Check sheet for the modelled part. Datum: model origin and axes. Units: mm. Face numbers are marked on the shaded views. A direction names the side the tool comes from. Round coordinates to 2 decimals unless told otherwise and drop trailing zeros. Write each loop counter-clockwise with the first axis right and the second up, starting at its lowest first coordinate (ties: lowest second). Pieces come first, ordered by that corner, then holes. Notation, with made-up numbers: (77, -28.5) -> (128, -28.5) arc R6 cw to (128, -17.5) -> close; hole circle Ø7 at (-38, -39). An arc over 180 degrees is marked (long way). Write item = value, one per line.
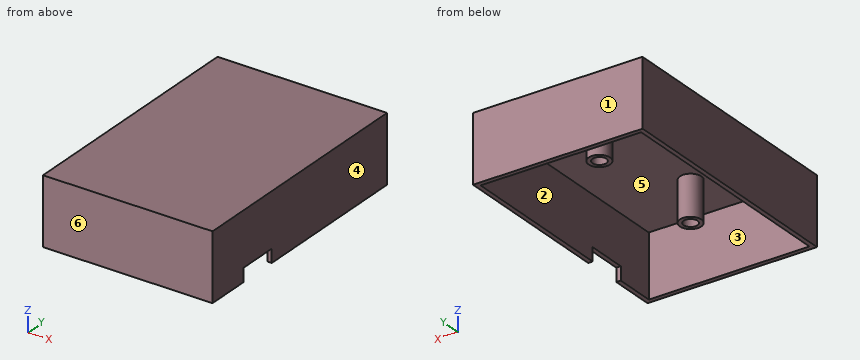
from build123d import *

# Parameters (mm, degrees)
SKETCH030_W     = 38
SKETCH030_H     = 56
PAD017_DEPTH    = 15
SKETCH031_W     = 36
SKETCH031_H     = 54
POCKET007_DEPTH = 14
SKETCH033_R     = 2.4
SKETCH033_R_2   = 1.55
PAD019_DEPTH    = 9
SKETCH038_W     = 9
SKETCH038_H     = 3
POCKET010_DEPTH = 5


with BuildPart() as part:
    # Sketch030 → Pad017 (new body)
    with BuildSketch(Plane.XY):
        Rectangle(SKETCH030_W, SKETCH030_H)
    extrude(amount=PAD017_DEPTH)

    # Sketch031 (on Face5 of Pad017) → Pocket007 (cut)
    with BuildSketch(Plane(origin=(0, 0, 0), x_dir=(1, 0, 0), z_dir=(0, 0, -1))):
        Rectangle(SKETCH031_W, SKETCH031_H)
    extrude(amount=-POCKET007_DEPTH, mode=Mode.SUBTRACT)

    # Sketch033 (on Face11 of Pocket007) → Pad019 (join)
    with BuildSketch(Plane(origin=(0, 0, 14), x_dir=(1, 0, 0), z_dir=(0, 0, -1))):
        with Locations((0, 14.65)):
            Circle(SKETCH033_R)
        with Locations((0, 14.65)):
            Circle(SKETCH033_R_2, mode=Mode.SUBTRACT)
    pad019 = extrude(amount=PAD019_DEPTH)

    # Mirrored009: Pad019 across XZ
    add(pad019.mirror(Plane.XZ))

    # Sketch038 (on Face3 of Mirrored009) → Pocket010 (cut)
    with BuildSketch(Plane.YZ.offset(19)):
        with Locations((-13.5, 1.5)):
            Rectangle(SKETCH038_W, SKETCH038_H)
    extrude(amount=-POCKET010_DEPTH, mode=Mode.SUBTRACT)


with BuildPart() as part_1:
    # Body007 placement: moved
    add(part.part.moved(Location((0, 0, 6.6))))


solid = part_1.part
(1) Release check for a two-part mould opening along X. For the marked faces 3, 4, 5 and 6 record: pulls with the +X half, pulls with the -X half, needs draft (parallel to the pull), parting line crosses it, or undercut.
Worked answers:
face_3 = undercut
face_4 = pulls with the +X half
face_5 = undercut
face_6 = needs draft
(2) Sectioned sample at D-D on x = 0. Enter the section's corners in (y, z).
Worked answers:
outline = (-28, 6.6) -> (-27, 6.6) -> (-27, 20.6) -> (-17.05, 20.6) -> (-17.05, 11.6) -> (-16.2, 11.6) -> (-16.2, 20.6) -> (-13.1, 20.6) -> (-13.1, 11.6) -> (-12.25, 11.6) -> (-12.25, 20.6) -> (12.25, 20.6) -> (12.25, 11.6) -> (13.1, 11.6) -> (13.1, 20.6) -> (16.2, 20.6) -> (16.2, 11.6) -> (17.05, 11.6) -> (17.05, 20.6) -> (27, 20.6) -> (27, 6.6) -> (28, 6.6) -> (28, 21.6) -> (-28, 21.6) -> close
(3) Sectioned sample at B-B on y = -10.5. Enter the section's corners in (x, z).
Worked answers:
outline = (-19, 6.6) -> (-18, 6.6) -> (-18, 20.6) -> (18, 20.6) -> (18, 9.6) -> (19, 9.6) -> (19, 21.6) -> (-19, 21.6) -> close
(4) Material ranges on L1, parallel to Y at x = 0, z = 14.5; L2, parallel to X at y = -14.65, z = 15.5; L3, parallel to Y at x = 2.5, z = 12.25, recorded low to high. Write a range as [from, to].
Worked answers:
L1 = [-28, -27], [-17.05, -16.2], [-13.1, -12.25], [12.25, 13.1], [16.2, 17.05], [27, 28]
L2 = [-19, -18], [-2.4, -1.55], [1.55, 2.4], [18, 19]
L3 = [-28, -27], [27, 28]
(5) Access from +Z, -Z, +X, -X, +Y, -Y to the whole of each face (thin tool, end or side, straight path). Record for the marked faces 1 and 2.
Worked answers:
face_1 = +Z, -Z, +X, -X, +Y
face_2 = -Z
(6) Sectioned sample at C-C on z = 8. Enter the section's corners in (x, y), then the cut area to 3 significant figures.
Worked answers:
outline = (-19, -28) -> (19, -28) -> (19, -18) -> (18, -18) -> (18, -27) -> (-18, -27) -> (-18, 27) -> (18, 27) -> (18, -9) -> (19, -9) -> (19, 28) -> (-19, 28) -> close
area = 175 mm²
(7) Sectioned sample at A-A on z = 14. Enter the section's corners in (x, y).
Worked answers:
outline = (-19, -28) -> (19, -28) -> (19, 28) -> (-19, 28) -> close; circle Ø4.8 at (0, -14.65); circle Ø4.8 at (0, 14.65); hole (-18, -27) -> (18, -27) -> (18, 27) -> (-18, 27) -> close; hole circle Ø3.1 at (0, -14.65); hole circle Ø3.1 at (0, 14.65)
(8) Go/stop test with flat-tipped pins: P1, Ø4, axis at x = -0.5, y = 15.5, coming from the -Z side; P2, Ø2.5, axis at x = 0, y = -14.65, coming from the -Z side; P3, Ø0.5, axis at x = 18.5, y = -14.5, coming from the -Z side. Record where each tip stops, or that it passes through.
Worked answers:
P1 = 11.6
P2 = 20.6
P3 = 9.6
